```python
from build123d import *

# Parameters (mm, degrees)
M6X1_0_TAPPED_HOLE1_D     = 5
M6X1_0_TAPPED_HOLE1_DEPTH = 12.99972
M6X1_0_TAPPED_HOLE1_TIP   = 1.502151548
SKETCH4_R                 = 1.25
CUT_EXTRUDE1_DEPTH        = 12.7


with BuildPart() as part:
    # Sketch1 → Revolve1 (revolve)
    with BuildSketch(Plane(origin=(0, 0, 0), x_dir=(0, 0, -1), z_dir=(1, 0, 0)), mode=Mode.PRIVATE) as revolve1_sk:
        with BuildLine():
            Line((-15, 0), (0, 0))
            Line((0, 0), (0, 6.4997425))
            ThreePointArc((0, 6.4997425), (-6.51425993, 5.756273724), (-12.71143042, 3.615384615))
            ThreePointArc((-12.71143042, 3.615384615), (-14.379772306, 2.13942496), (-15, 0))
        make_face()
    revolve(revolve1_sk.sketch.rotate(Axis((0, 0, 0), (0, 0, 1)), 90), axis=Axis((0, 0, 0), (0, 0, 1)))

    # M6x1.0 Tapped Hole1
    with Locations(Plane(origin=(0, 0, 0), x_dir=(-1, 0, 0), z_dir=(0, 0, -1))):
        with Locations((0, 0)):
            Hole(M6X1_0_TAPPED_HOLE1_D / 2, depth=M6X1_0_TAPPED_HOLE1_DEPTH)
            with Locations((0, 0, -(M6X1_0_TAPPED_HOLE1_DEPTH + M6X1_0_TAPPED_HOLE1_TIP / 2))):  # 118° drill point
                Cone(0, M6X1_0_TAPPED_HOLE1_D / 2, M6X1_0_TAPPED_HOLE1_TIP, mode=Mode.SUBTRACT)

    # Sketch4 → Cut-Extrude1 (cut, symmetric)
    with BuildSketch(Plane(origin=(0, 0, 0), x_dir=(0, 0, -1), z_dir=(1, 0, 0))):
        with Locations(Location((-12, 0, 0), (0, 0, 290.171984379))):
            Circle(SKETCH4_R)
    extrude(amount=CUT_EXTRUDE1_DEPTH, both=True, mode=Mode.SUBTRACT)


solid = part.part
```
CAD build for the part. Positions are in the model's coordinates, mm. A direction names the side the tool comes from. Round coordinates to 2 decimals unless told otherwise and drop trailing zeros. Return JSON: item names as keys, results as strings. Group by question number.
Item 1: Flat gauge pins, fed straight in: pin 1 Ø4 at (x, z) = (2.5, 8) entering from -Y; pin 2 Ø1.5 at (x, z) = (0, 5) entering from -Y; pin 3 Ø1 at (x, z) = (3.5, 7.5) entering from -Y. Where does each tip first touch, or does it go through?
Item 2: 3-axis set-ups, long thin cutter, end or side, ignore diameter. For faces 1 (the face through (2.385, 0.751, 6.591)), 2 (the face through (3.027, 0.58, 10.893)): which of +Z, -Z, +X, -X, +Y, -Y reach the whole face in a straight line?
Item 3: Probe probe 1 along X at (y, z) = (1.5, 8); probe 2 along Y at (x, z) = (1.75, 10.5); probe 3 along Y at (x, z) = (0, 3.5). List the from-to ranges inside material, lowest first.
Item 4: Mould opens along Y. For faces 3 (the face through (-2.99, -0.27, 10.78)), 4 (the face through (3, 0, 0)) say: +Y half, -Y half, draft (parallel to the pull), parting line (faces both ways), or undercut.
Resolved:
{
 "1": {"pin 1": "stops at y = -5.64", "pin 2": "stops at y = -6.18", "pin 3": "stops at y = -4.66"},
 "2": {"face 1": "-Z", "face 2": "+X, -X"},
 "3": {"probe 1": "x = -5.17 to -2, 2 to 5.17", "probe 2": "y = -4.21 to -1.79, 1.79 to 4.21", "probe 3": "y = -6.28 to -2.5, 2.5 to 6.28"},
 "4": {"face 3": "undercut", "face 4": "draft"}
}
